```python
from build123d import *

# Parameters (mm, degrees)
SKETCH1_R               = 22.5
BOSS_EXTRUDE1_DEPTH     = 15
SKETCH2_R               = 20.25
SKETCH2_R_2             = 18.5
BOSS_EXTRUDE2_DEPTH     = 10
CUT_EXTRUDE1_DEPTH      = 41.466035141
CUT_EXTRUDE1_DEPTH_BACK = 41.466035141
SKETCH4_W               = 10
SKETCH4_H               = 24.752073401
FILLET1_R               = 0.8
SKETCH5_R               = 20.25
SKETCH5_R_2             = 12.5
CUT_EXTRUDE2_DEPTH      = 10


with BuildPart() as part:
    # Sketch1 → Boss-Extrude1 (new body)
    with BuildSketch(Plane.XY):
        Circle(SKETCH1_R)
    extrude(amount=BOSS_EXTRUDE1_DEPTH)

    # Sketch2 → Boss-Extrude2 (add)
    with BuildSketch(Plane.XY.offset(15)):
        Circle(SKETCH2_R)
        Circle(SKETCH2_R_2, mode=Mode.SUBTRACT)
    extrude(amount=BOSS_EXTRUDE2_DEPTH)

    # Sketch4 → Cut-Extrude1 (cut, two sides: drawn at the far end of the back side and taken through both)
    with BuildSketch(Plane(origin=(0, 0, 0), x_dir=(0, 0, -1), z_dir=(1, 0, 0)).offset(-CUT_EXTRUDE1_DEPTH_BACK)):
        with Locations((-20, 12.376036701)):
            Rectangle(SKETCH4_W, SKETCH4_H)
    extrude(amount=CUT_EXTRUDE1_DEPTH + CUT_EXTRUDE1_DEPTH_BACK, mode=Mode.SUBTRACT)

    # Fillet1
    fillet1_edges = [part.edges().sort_by_distance(p)[0] for p in [
        (-22.5, 0, 0),
        (-22.5, 0, 15),
    ]]
    fillet(fillet1_edges, radius=FILLET1_R)

    # Sketch5 → Cut-Extrude2 (cut)
    with BuildSketch(Plane(origin=(0, 0, 0), x_dir=(-1, 0, 0), z_dir=(0, 0, -1))):
        Circle(SKETCH5_R)
        Circle(SKETCH5_R_2, mode=Mode.SUBTRACT)
    extrude(amount=-CUT_EXTRUDE2_DEPTH, mode=Mode.SUBTRACT)


solid = part.part
```
Geometry check sheet. Reference: the model listing, model coordinates, mm. A direction names the side the tool comes from. Give positions to 0.01 mm unless a question says otherwise; leave off trailing zeros. Write each loop counter-clockwise with the first axis right and the second up, starting at its lowest first coordinate (ties: lowest second). Pieces come first, ordered by that corner, then holes. Notation, with made-up numbers: (14, 44.25) - (30, 44.25) arc R31 cw to (30, 77.25) - close; hole circle Ø10 at (-9.5, 21). An arc over 180 degrees is marked (long way). Use a Markdown table: item, result.
Q1. Go/stop test with flat-tipped pins: P1, Ø3, axis at x = 15, z = 6, coming from the +Y side; P2, Ø6, axis at y = -7.5, z = 16.5, coming from the +X side; P3, Ø4, axis at x = 13.5, y = -2.5, coming from the -Z side; P4, Ø1.9, axis at x = -19.5, z = 22, coming from the +Y side. Record where each tip stops, or that it passes through.
Computed:
| item | result |
|---|---|
| P1 | stops at y = 18 |
| P2 | stops at x = 21.83 |
| P3 | stops at z = 0 |
| P4 | stops at y = 0 |
Q2. Thickness scan on L1, parallel to Y at x = 0, z = 7; L2, parallel to X at y = -5.5, z = 4.75; L3, parallel to X at y = -7, z = 4.25. Record the ranges inside material, lowest first. Write a range as [from, to].
Computed:
| item | result |
|---|---|
| L1 | y = [-22.5, -20.25], [-12.5, 12.5], [20.25, 22.5] |
| L2 | x = [-21.82, -19.49], [-11.22, 11.22], [19.49, 21.82] |
| L3 | x = [-21.38, -19], [-10.36, 10.36], [19, 21.38] |
Q3. Draft check along Y on faces 1 (the face through (19, 0, 20)), 2 (the face through (-11.923, 3.755, 4.93)), 3 (the face through (10.382, -19.961, 7.406)). Enter one of: pulls with the +Y half, pulls with the -Y half, needs draft (parallel to the pull), parting line crosses it, or undercut.
Computed:
| item | result |
|---|---|
| face 1 | pulls with the +Y half |
| face 2 | undercut |
| face 3 | parting line crosses it |
Q4. Set-up check for faces 4 (the face through (-19, 0, 20)), 5 (the face through (-0.407, -18.496, 19.93)), 6 (the face through (-0.445, -20.245, 19.93)), 7 (the face through (-11, 17, 5)): record each of +Z, -Z, +X, -X, +Y, -Y from which the full face is reachable in a straight line by a thin tool's end or side.
Computed:
| item | result |
|---|---|
| face 4 | +Z, +X, -X, +Y |
| face 5 | +Z, +Y |
| face 6 | +Z, -Y |
| face 7 | -Z |
Q5. Section check A-A, the plane z = 6.5. Enter the section's corners in (x, y).
Computed:
| item | result |
|---|---|
| outline | circle Ø45 at (0, 0); circle Ø25 at (0, 0); hole circle Ø40.5 at (0, 0) |
Q6. Section check B-B, the plane x = 0. Enter the section's corners in (y, z).
Computed:
| item | result |
|---|---|
| outline | (-22.5, 0.8) arc R0.8 ccw to (-21.7, 0) - (-20.25, 0) - (-20.25, 10) - (-12.5, 10) - (-12.5, 0) - (12.5, 0) - (12.5, 10) - (20.25, 10) - (20.25, 0) - (21.7, 0) arc R0.8 ccw to (22.5, 0.8) - (22.5, 14.2) arc R0.8 ccw to (21.7, 15) - (-18.5, 15) - (-18.5, 25) - (-20.25, 25) - (-20.25, 15) - (-21.7, 15) arc R0.8 ccw to (-22.5, 14.2) - close |
Q7. Section check C-C, the plane z = 19.75. Enter the section's corners in (x, y).
Computed:
| item | result |
|---|---|
| outline | (-20.25, 0) arc R20.25 ccw to (20.25, 0) - (18.5, 0) arc R18.5 cw to (-18.5, 0) - close |
